Check sheet for the modelled part. Datum: model origin and axes. Units: mm. Face numbers are marked on the shaded views. A direction names the side the tool comes from. Give positions to 0.01 mm unless a question says otherwise; leave off trailing zeros. Loops run counter-clockwise (first coordinate to the right, second up) from the corner with the lowest first, then second, coordinate; pieces in that order, holes last. Notation, with made-up numbers: (57, 17) -> (81, 17) arc R23 ccw to (81, 33) -> close; hole circle Ø5 at (-33.5, 72). An arc over 180 degrees is marked (long way). Answer as CSV lines item,"result". Start each with the question number.
(1) Access from +Z, -Z, +X, -X, +Y, -Y to the whole of each face (thin tool, end or side, straight path). Record for the marked faces 5, 6, 7, 8 and 9.
(2) Material ranges on line 1 (Y direction, x = 0, z = 9.8); line 2 (Y direction, x = 0, z = 11.7); line 3 (Y direction, x = 17.5, z = 10), recorded low to high. Write a range as from..to.
(3) Section check B-B on y = 14. Enter the section's corners in (x, z), plus the area to 3 significant figures.
(4) Section check A-A on x = 14.5. Enter the section's corners in (y, z).
(5) Section check D-D on x = -21.5. Enter the section's corners in (y, z), plus the area to 3 significant figures.
(6) Section check C-C on z = 9. Enter the section's corners in (x, y).
(7) Gauge pin test, flat ends, axial feed: pin 1 Ø3 at (x, z) = (-4.5, 9) entering from +Y; pin 2 Ø8 at (y, z) = (-23.5, 3) entering from -X; pin 3 Ø3 at (x, z) = (8.5, 11.5) entering from +Y; pin 4 Ø1.5 at (x, y) = (1.5, 2) entering from -Z. Record the tip position at first contact, or that the pin passes through.
(8) Release check for a two-part mould opening along Y. For the marked faces 1, 2, 3 and 4 record: pulls with the +Y half, pulls with the -Y half, needs draft (parallel to the pull), parting line crosses it, or undercut.
Autodesk Inventor part; units mm, degrees
ref_plane "YZ Plane" through (0, 0, 0) normal (1, 0, 0) x (0, 1, 0)
ref_plane "XZ Plane" through (0, 0, 0) normal (0, 1, 0) x (-1, 0, 0)
ref_plane "XY Plane" through (0, 0, 0) normal (0, 0, 1) x (1, 0, 0)
sketch "Szkic1" plane through (0, 0, 0) normal (0, 0, 1) x (1, 0, 0)
  line L0 (-20.4343, -10) -> (-41.564, -10)
  line L1 (-20.4343, 10) -> (-41.564, 10)
  line L2 (-10, -20.4343) -> (-10, -41.564)
  line L3 (10, -20.4343) -> (10, -41.564)
  line L4 (20.4343, -10) -> (41.564, -10)
  line L5 (20.4343, 10) -> (41.564, 10)
  line L6 (10, 20.4343) -> (10, 41.564)
  line L7 (-10, 20.4343) -> (-10, 41.564)
  arc A0 (-36.4014, 10) -> (-36.4014, -10) centre (0, 0) ccw
  arc A1 (-31.1859, 10) -> (-31.1859, -10) centre (0, 0) ccw
  arc A2 (-28.019, 10) -> (-28.019, -10) centre (0, 0) ccw
  arc A3 (-24.8105, 10) -> (-24.8105, -10) centre (0, 0) ccw
  arc A4 (-23.7289, 10) -> (-23.7289, -10) centre (0, 0) ccw
  arc A5 (-20.4343, 10) -> (-20.4343, -10) centre (0, 0) ccw
  arc A6 (-41.564, 10) -> (-41.564, -10) centre (0, 0) ccw
  arc A7 (-10, -20.4343) -> (10, -20.4343) centre (0, 0) ccw
  arc A8 (-10, -23.7289) -> (10, -23.7289) centre (0, 0) ccw
  arc A9 (-10, -24.8105) -> (10, -24.8105) centre (0, 0) ccw
  arc A10 (-10, -28.019) -> (10, -28.019) centre (0, 0) ccw
  arc A11 (-10, -31.1859) -> (10, -31.1859) centre (0, 0) ccw
  arc A12 (-10, -36.4014) -> (10, -36.4014) centre (0, 0) ccw
  arc A13 (-10, -41.564) -> (10, -41.564) centre (0, 0) ccw
  arc A14 (20.4343, -10) -> (20.4343, 10) centre (0, 0) ccw
  arc A15 (10, 20.4343) -> (-10, 20.4343) centre (0, 0) ccw
  arc A16 (23.7289, -10) -> (23.7289, 10) centre (0, 0) ccw
  arc A17 (10, 23.7289) -> (-10, 23.7289) centre (0, 0) ccw
  arc A18 (24.8105, -10) -> (24.8105, 10) centre (0, 0) ccw
  arc A19 (10, 24.8105) -> (-10, 24.8105) centre (0, 0) ccw
  arc A20 (28.019, -10) -> (28.019, 10) centre (0, 0) ccw
  arc A21 (10, 28.019) -> (-10, 28.019) centre (0, 0) ccw
  arc A22 (31.1859, -10) -> (31.1859, 10) centre (0, 0) ccw
  arc A23 (10, 31.1859) -> (-10, 31.1859) centre (0, 0) ccw
  arc A24 (36.4014, -10) -> (36.4014, 10) centre (0, 0) ccw
  arc A25 (10, 36.4014) -> (-10, 36.4014) centre (0, 0) ccw
  arc A26 (41.564, -10) -> (41.564, 10) centre (0, 0) ccw
  arc A27 (10, 41.564) -> (-10, 41.564) centre (0, 0) ccw
  circle A28 centre (0, 0) radius 4.5
  circle A29 centre (0, 0) radius 19.75
  line L8 (10, 20.4343) -> (10, 17.0312)
  line L9 (-10, 20.4343) -> (-10, 17.0312)
  line L10 (10, -20.4343) -> (10, -17.0312)
  line L11 (-20.4343, -10) -> (-17.0312, -10)
  line L12 (-20.4343, 10) -> (-17.0312, 10)
  line L13 (-10, -17.0312) -> (-10, -20.4343)
  line L14 (20.4343, 10) -> (17.0312, 10)
  line L15 (20.4343, -10) -> (17.0312, -10)
  line L16 (0, -4.5265) -> (0, 3.8342)
  line L17 (3.7027, 0) -> (-4.6541, 0)
  arc A30 (0, -14) -> (14, 0) centre (0, 0) ccw construction
  arc A31 (0, -16.5) -> (16.5, 0) centre (0, 0) ccw
  arc A32 (0, -11.5) -> (11.5, 0) centre (0, 0) ccw
  arc A33 (0, -11.5) -> (0, -16.5) centre (0, -14) ccw
  arc A34 (16.5, 0) -> (11.5, 0) centre (14, 0) ccw
  arc A35 (0, 14) -> (-14, 0) centre (0, 0) ccw construction
  arc A36 (0, 16.5) -> (-16.5, 0) centre (0, 0) ccw
  arc A37 (0, 11.5) -> (-11.5, 0) centre (0, 0) ccw
  arc A38 (0, 11.5) -> (0, 16.5) centre (0, 14) ccw
  arc A39 (-16.5, 0) -> (-11.5, 0) centre (-14, 0) ccw
  arc A40 (0, -12) -> (12, 0) centre (0, 0) ccw
  arc A41 (0, -12) -> (0, -16) centre (0, -14) ccw
  arc A42 (0, -16) -> (16, 0) centre (0, 0) ccw
  arc A43 (16, 0) -> (12, 0) centre (14, 0) ccw
  arc A44 (0, 12) -> (-12, 0) centre (0, 0) ccw
  arc A45 (0, 12) -> (0, 16) centre (0, 14) ccw
  arc A46 (0, 16) -> (-16, 0) centre (0, 0) ccw
  arc A47 (-16, 0) -> (-12, 0) centre (-14, 0) ccw
  point P0 (10, -17.0312)
  point P1 (-10, -17.0312)
  point P2 (-10, 17.0312)
  dimension "d62" = 22.75
  dimension "d14" = 9
  dimension "d42" = 14
  dimension "d43" = 14
  dimension "d44" = 14
  dimension "d45" = 14
  dimension "d47" = 5
  dimension "d48" = 5
  dimension "d57" = 0.5
  dimension "d58" = 0.5
extrude "Wyciągnięcie proste2" add sketch "Szkic1" along normal blind 14 contours L0 A4 L1 A5 | A5 L12 A29 L11 | L0 A3 L1 A4 | A29 | L0 A2 L1 A3 | A29 L10 A7 L13 | L0 A1 L1 A2 | L9 A15 L8 A29 | A7 L3 A8 L2 | L0 A0 L1 A1 | L7 A17 L6 A15 | A29 L14 A14 L15 | A8 L3 A9 L2 | L0 A6 L1 A0 | L7 A19 L6 A17 | A14 L5 A16 L4 | A9 L3 A10 L2 | L7 A21 L6 A19 | A16 L5 A18 L4 | A10 L3 A11 L2 | L7 A23 L6 A21 | A18 L5 A20 L4 | A11 L3 A12 L2 | L7 A25 L6 A23 | A20 L5 A22 L4 | A12 L3 A13 L2 | L7 A27 L6 A25 | A22 L5 A24 L4 | A24 L5 A26 L4 | A33 A32 A34 A31 | A38 A37 A39 A36 | A40 A43 A42 A41 | A44 A47 A46 A45
extrude "Wyciągnięcie proste3" cut sketch "Szkic1" along normal blind 2 contours A5 L12 A29 L11 | A29 L10 A7 L13 | L9 A15 L8 A29 | A29 L14 A14 L15
extrude "Wyciągnięcie proste4" cut sketch "Szkic1" along normal blind 4 contours L0 A4 L1 A5 | A7 L3 A8 L2 | L7 A17 L6 A15 | A14 L5 A16 L4
extrude "Wyciągnięcie proste5" cut sketch "Szkic1" along normal blind 6 contours L0 A3 L1 A4 | A8 L3 A9 L2 | L7 A19 L6 A17 | A16 L5 A18 L4
extrude "Wyciągnięcie proste6" cut sketch "Szkic1" along normal blind 8 contours L0 A2 L1 A3 | A9 L3 A10 L2 | L7 A21 L6 A19 | A18 L5 A20 L4
extrude "Wyciągnięcie proste7" cut sketch "Szkic1" along normal blind 10 contours L0 A1 L1 A2 | A10 L3 A11 L2 | L7 A23 L6 A21 | A20 L5 A22 L4
extrude "Wyciągnięcie proste8" cut sketch "Szkic1" along normal blind 12 contours L0 A0 L1 A1 | A11 L3 A12 L2 | L7 A25 L6 A23 | A22 L5 A24 L4
extrude "Wyciągnięcie proste9" cut sketch "Szkic1" along normal blind 15 contours L0 A6 L1 A0 | A12 L3 A13 L2 | L7 A27 L6 A25 | A24 L5 A26 L4
sketch "Szkic2" plane through (0, 0, 14) normal (0, 0, 1) x (1, 0, 0)
  circle A0 centre (0, 0) radius 4.5
  line L0 (10, -36.4014) -> (10, -17.0312)
  arc A1 (10, -17.0312) -> (17.0312, -10) centre (0, 0) ccw
  line L1 (17.0312, -10) -> (36.4014, -10)
  line L2 (36.4014, 10) -> (17.0312, 10)
  arc A2 (17.0312, 10) -> (10, 17.0312) centre (0, 0) ccw
  line L3 (10, 17.0312) -> (10, 36.4014)
  line L4 (-10, 36.4014) -> (-10, 17.0312)
  arc A3 (-10, 17.0312) -> (-17.0312, 10) centre (0, 0) ccw
  line L5 (-17.0312, 10) -> (-36.4014, 10)
  line L6 (-36.4014, -10) -> (-17.0312, -10)
  arc A4 (-17.0312, -10) -> (-10, -17.0312) centre (0, 0) ccw
  line L7 (-10, -17.0312) -> (-10, -36.4014)
  circle A5 centre (0, 0) radius 9.5
  arc A6 (36.4014, -10) -> (36.4014, 10) centre (0, 0) ccw
  arc A7 (10, 36.4014) -> (-10, 36.4014) centre (0, 0) ccw
  arc A8 (-36.4014, 10) -> (-36.4014, -10) centre (0, 0) ccw
  arc A9 (-10, -36.4014) -> (10, -36.4014) centre (0, 0) ccw
  dimension "d33" = 19
extrude "Wyciągnięcie proste10" cut sketch "Szkic2" against normal blind 6 contours A5
chamfer "Faza2" distance 1 angle 45 1 edges at (-4.5, 0, 0)
extrude "Wyciągnięcie proste12" cut sketch "Szkic1" along normal blind 17 contours A40 A43 A42 A41 | A44 A47 A46 A45
properties part number "3DP_ABS_Filament_Spool_Mount_Bearing_Block"
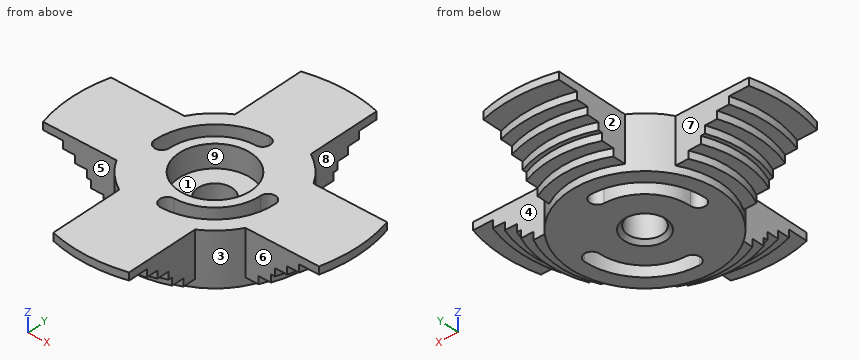
Working result:
1,face 5,"+Z, -Z, -X, -Y"
1,face 6,"+Z, -Z, +X, -Y"
1,face 7,"+Z, -Z, -X, +Y"
1,face 8,"+Z, -Z, +X, +Y"
1,face 9,"+Z"
2,line 1,"y = -29.75..-16, -12..-9.5, 9.5..12, 16..29.75"
2,line 2,"y = -32.75..-16, -12..-9.5, 9.5..12, 16..32.75"
2,line 3,"y = -10..10"
3,outline,"(-13.93, 0) -> (-7.75, 0) -> (-7.75, 14) -> (-13.93, 14) -> close; (2, 0) -> (13.93, 0) -> (13.93, 14) -> (2, 14) -> close"
3,area,"254 mm^2"
4,outline,"(-13.41, 0) -> (-6.76, 0) -> (-6.76, 14) -> (-13.41, 14) -> close; (1.94, 0) -> (13.41, 0) -> (13.41, 14) -> (1.94, 14) -> close"
5,outline,"(-10, 4) -> (-7.44, 4) -> (-7.44, 2) -> (7.44, 2) -> (7.44, 4) -> (10, 4) -> (10, 14) -> (-10, 14) -> close"
5,area,"230 mm^2"
6,outline,"(-28.02, -10) -> (-17.03, -10) arc R19.75 ccw to (-10, -17.03) -> (-10, -28.02) arc R29.75 ccw to (10, -28.02) -> (10, -17.03) arc R19.75 ccw to (17.03, -10) -> (28.02, -10) arc R29.75 ccw to (28.02, 10) -> (17.03, 10) arc R19.75 ccw to (10, 17.03) -> (10, 28.02) arc R29.75 ccw to (-10, 28.02) -> (-10, 17.03) arc R19.75 ccw to (-17.03, 10) -> (-28.02, 10) arc R29.75 ccw to start; hole (-16, 0) arc R2 ccw to (-12, 0) arc R12 cw to (0, 12) arc R2 ccw to (0, 16) arc R16 ccw to start; hole circle Ø19 at (0, 0); hole (0, -16) arc R16 ccw to (16, 0) arc R2 ccw to (12, 0) arc R12 cw to (0, -12) arc R2 ccw to start"
7,pin 1,"stops at y = 32.57"
7,pin 2,"stops at x = -10"
7,pin 3,"stops at y = 37.08"
7,pin 4,"passes through"
8,face 1,"undercut"
8,face 2,"needs draft"
8,face 3,"parting line crosses it"
8,face 4,"pulls with the +Y half"
